Here's how the part is built. I have some questions about the finished solid (model axes, mm). A direction names the side the tool comes from. Coordinates: 2 decimals unless noted, no trailing zeros. Loops run counter-clockwise (first coordinate to the right, second up) from the corner with the lowest first, then second, coordinate; pieces in that order, holes last. Notation, with made-up numbers: (-5.75, 18) -> (39.25, 18) arc R18 ccw to (39.25, 41) -> close; hole circle Ø3 at (62.5, -33). An arc over 180 degrees is marked (long way). Use CSV: the item, a comma, the result in double quotes. Start each with the question number.
from build123d import *

# Parameters (mm, degrees)
SKETCH1_R           = 25
SKETCH1_W           = 27.5
SKETCH1_H           = 27.5
BOSS_EXTRUDE1_DEPTH = 55
BOSS_EXTRUDE2_START = 5
SKETCH2_R           = 25
SKETCH2_W           = 27.5
SKETCH2_H           = 27.5
BOSS_EXTRUDE2_DEPTH = 5
SKETCH3_W           = 25
SKETCH3_H           = 50
BOSS_EXTRUDE3_DEPTH = 80
FILLET1_R           = 2.5
FILLET2_R           = 2.5
SKETCH21_W          = 54.3
SKETCH21_H          = 20.3
CUT_EXTRUDE1_DEPTH  = 11.3
SKETCH22_W          = 40.3
SKETCH22_H          = 20.3
CUT_EXTRUDE2_DEPTH  = 93.059763198
CUT_EXTRUDE3_DEPTH  = 88.464278423
SKETCH23_R          = 2.15
CUT_EXTRUDE4_DEPTH  = 93.059763198
CUT_EXTRUDE7_DEPTH  = 27.5


with BuildPart() as part:
    # Sketch1 → Boss-Extrude1 (new body)
    with BuildSketch(Plane.XY):
        Circle(SKETCH1_R)
        Rectangle(SKETCH1_W, SKETCH1_H, mode=Mode.SUBTRACT)
    extrude(amount=BOSS_EXTRUDE1_DEPTH)

    # Sketch2 → Boss-Extrude2 (add)
    # profile 1 of 2: a face of its own
    with BuildSketch(Plane(origin=(0, 0, 0), x_dir=(-1, 0, 0), z_dir=(0, 0, -1)).offset(BOSS_EXTRUDE2_START)):
        Circle(SKETCH2_R)
        Rectangle(SKETCH2_W, SKETCH2_H, mode=Mode.SUBTRACT)
    # profile 2 of 2: a face of its own
    with BuildSketch(Plane(origin=(0, 0, 0), x_dir=(-1, 0, 0), z_dir=(0, 0, -1)).offset(BOSS_EXTRUDE2_START)):
        Rectangle(SKETCH2_W, SKETCH2_H)
    extrude(amount=-BOSS_EXTRUDE2_DEPTH)

    # Sketch3 → Boss-Extrude3 (add)
    with BuildSketch(Plane(origin=(0, 0, -5), x_dir=(-1, 0, 0), z_dir=(0, 0, -1))):
        with Locations((12.5, 0)):
            Rectangle(SKETCH3_W, SKETCH3_H)
    extrude(amount=BOSS_EXTRUDE3_DEPTH)

    # Fillet1
    fillet1_edges = [part.edges().sort_by_distance(p)[0] for p in [
        (-13.75, 13.75, 27.5),
        (-13.75, -13.75, 27.5),
        (13.75, -13.75, 27.5),
        (13.75, 13.75, 27.5),
    ]]
    fillet(fillet1_edges, radius=FILLET1_R)

    # Fillet2
    fillet2_edges = [part.edges().sort_by_distance(p)[0] for p in [
        (0, 13.75, 55),
        (-13.75, 0, 55),
        (0, -13.75, 55),
        (13.75, 0, 55),
        (-13.017766953, 13.017766953, 55),
        (-13.017766953, -13.017766953, 55),
        (13.017766953, -13.017766953, 55),
        (13.017766953, 13.017766953, 55),
    ]]
    fillet(fillet2_edges, radius=FILLET2_R)

    # Sketch21 → Cut-Extrude1 (cut)
    with BuildSketch(Plane(origin=(0, 0, 0), x_dir=(0, 0, -1), z_dir=(1, 0, 0))):
        with Locations((51.85, 0)):
            Rectangle(SKETCH21_W, SKETCH21_H)
    extrude(amount=-CUT_EXTRUDE1_DEPTH, mode=Mode.SUBTRACT)

    # Sketch22 → Cut-Extrude2 (cut, through all)
    with BuildSketch(Plane(origin=(0, 0, 0), x_dir=(0, 0, -1), z_dir=(1, 0, 0))):
        with Locations((51.7, 0)):
            Rectangle(SKETCH22_W, SKETCH22_H)
    extrude(amount=-CUT_EXTRUDE2_DEPTH, mode=Mode.SUBTRACT)

    # Sketch18 → Cut-Extrude3 (cut, through all)
    with BuildSketch(Plane.XY.offset(-5)):
        with BuildLine():
            Line((-25, -25), (0, -25))
            ThreePointArc((0, -25), (-17.67766953, -17.67766953), (-25, 0))
            Line((-25, 0), (-25, -25))
        make_face()
        with BuildLine():
            Line((-25, 25), (-25, 0))
            ThreePointArc((-25, 0), (-17.67766953, 17.67766953), (0, 25))
            Line((0, 25), (-25, 25))
        make_face()
    extrude(amount=-CUT_EXTRUDE3_DEPTH, mode=Mode.SUBTRACT)

    # Sketch23 → Cut-Extrude4 (cut, through all)
    with BuildSketch(Plane(origin=(0, 0, 0), x_dir=(0, 0, -1), z_dir=(1, 0, 0))):
        with Locations(Location((27.85, -5.25, 0), (0, 0, 90))):
            Circle(SKETCH23_R)
        with Locations(Location((75.85, 5.25, 0), (0, 0, 90))):
            Circle(SKETCH23_R)
        with Locations(Location((75.85, -5.25, 0), (0, 0, 90))):
            Circle(SKETCH23_R)
        with Locations(Location((27.85, 5.25, 0), (0, 0, 90))):
            Circle(SKETCH23_R)
    extrude(amount=-CUT_EXTRUDE4_DEPTH, mode=Mode.SUBTRACT)

    # Sketch24 → Cut-Extrude7 (cut, symmetric)
    with BuildSketch(Plane(origin=(0, 0, -51.7), x_dir=(-1, 0, 0), z_dir=(0, 0, -1))):
        with BuildLine():
            Line((13.3, 10.15), (13.3, -10.15))
            Line((13.3, -10.15), (22.846826913, -10.15))
            ThreePointArc((22.846826913, -10.15), (25, 0), (22.846826913, 10.15))
            Line((22.846826913, 10.15), (13.3, 10.15))
        make_face()
    extrude(amount=CUT_EXTRUDE7_DEPTH, both=True, mode=Mode.SUBTRACT)


solid = part.part
1) For P1, Ø3.5, axis at x = -7.5, z = -75.5, coming from the -Y side; P2, Ø2, axis at x = -12.5, z = -44, coming from the +Y side; P3, Ø3, axis at x = -17.5, z = -57, coming from the +Y side, each with a flat end and sliding along its axis, tell me the tip position at first contact or that it passes through.
2) I want a section at A-A, the plane z = -27.85. Please give me the cut outline in (x, y), plus the area to 3 significant figures.
3) I want a section at D-D, the plane x = -7.5. Please give me the cut outline in (y, z), plus the area to 3 significant figures.
4) I want a section at C-C, the plane y = -5.25. State how many separate pieces and enclosed holes the cut face has, plus the area to 3 significant figures.
5) Thinking about a two-plate mould opening in Y: for faces 1 (the face through (-12.286, -6.956, -29.158)), 2 (the face through (10, 0, -5)), 3 (the face through (-13.037, -12.998, 26.618)), which applies, pulls with the +Y half, pulls with the -Y half, needs draft (parallel to the pull), parting line crosses it, or undercut?
6) Which directions (+Z, -Z, +X, -X, +Y, -Y) give clear straight access to the entire face, cutting with the end or side of a thin tool? Please do faces 4 (the face through (-12.29, -5.72, -77.95)), 5 (the face through (-19, 0, -24.2)), 6 (the face through (0, 0, 0)), 7 (the face through (-11.3, 0, -28)).
7) Please list where these lines run through material, in increasing order: L1, parallel to Z at x = -12, y = 5; L2, parallel to Z at x = -2.5, y = 2; L3, parallel to Y at x = -12, z = -27. Write a range as [from, to].
8) I want a section at B-B, the plane z = 3.5. Please give me the cut outline in (x, y), plus the area to 3 significant figures.
Return value:
1,P1,"stops at y = -24.33"
1,P2,"stops at y = 22.2"
1,P3,"stops at y = 19.21"
2,outline,"(-22.85, -10.15) arc R25 ccw to (0, -25) -> (0, -10.15) -> (-11.3, -10.15) -> (-11.3, -7.4) -> (-13.3, -7.4) -> (-13.3, -10.15) -> close; (-22.85, 10.15) -> (-13.3, 10.15) -> (-13.3, 7.4) -> (-11.3, 7.4) -> (-11.3, 10.15) -> (0, 10.15) -> (0, 25) arc R25 ccw to start; (-13.3, -3.1) -> (-11.3, -3.1) -> (-11.3, 3.1) -> (-13.3, 3.1) -> close"
2,area,"512 mm²"
3,outline,"(-23.85, -85) -> (23.85, -85) -> (23.85, 55) -> (16.25, 55) arc R2.5 ccw to (13.75, 52.5) -> (13.75, 0) -> (-13.75, 0) -> (-13.75, 52.5) arc R2.5 ccw to (-16.25, 55) -> (-23.85, 55) -> close; hole (-10.15, -79) -> (10.15, -79) -> (10.15, -24.7) -> (-10.15, -24.7) -> close"
3,area,"4,060 mm²"
4,separate pieces,"4"
4,enclosed holes,"0"
4,area,"2,050 mm²"
5,face 1,"undercut"
5,face 2,"needs draft"
5,face 3,"undercut"
6,face 4,"+X, -X"
6,face 5,"-X"
6,face 6,"+Z"
6,face 7,"+X"
7,L1,"z = [-85, -77.99], [-73.71, -71.85], [-31.55, -29.99], [-25.71, 0]"
7,L2,"z = [-85, -79], [-24.7, 0]"
7,L3,"y = [-21.93, -7.22], [-3.28, 3.28], [7.22, 21.93]"
8,outline,"circle Ø50 at (0, 0); hole (-13.75, -11.25) arc R2.5 ccw to (-11.25, -13.75) -> (11.25, -13.75) arc R2.5 ccw to (13.75, -11.25) -> (13.75, 11.25) arc R2.5 ccw to (11.25, 13.75) -> (-11.25, 13.75) arc R2.5 ccw to (-13.75, 11.25) -> close"
8,area,"1,210 mm²"
